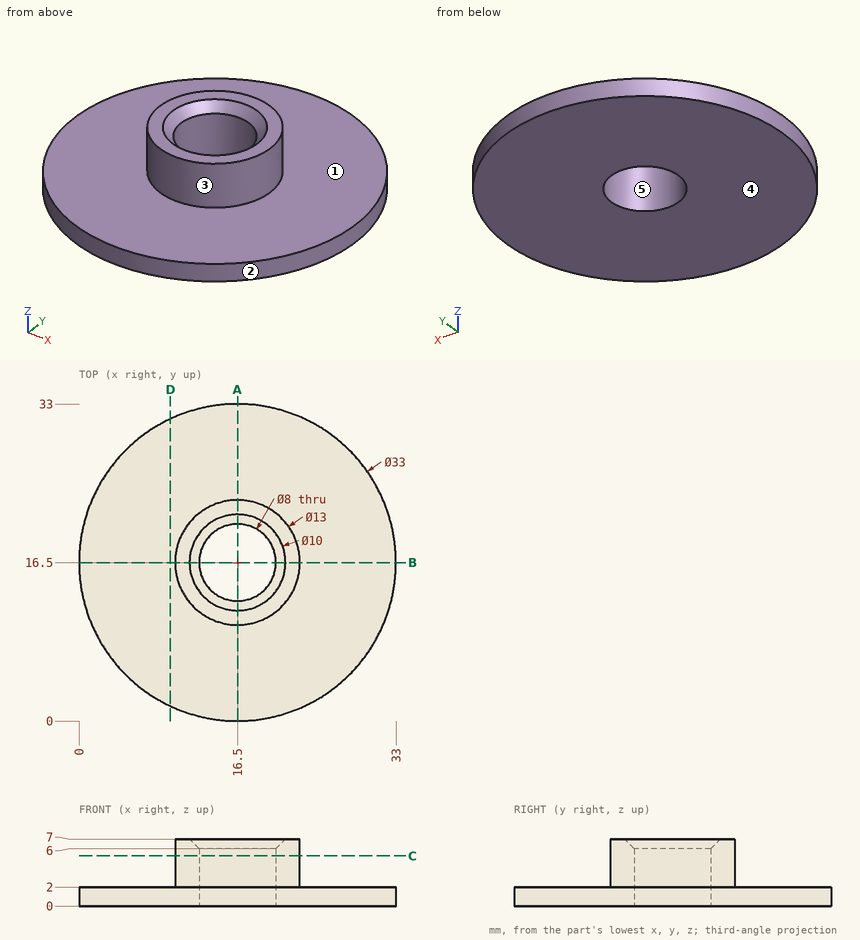
Here's the drawing with two shaded views (mm, measured from the low corner). I have some questions. A direction names the side the tool comes from. Give positions to 0.01 mm unless a question says otherwise; leave off trailing zeros. Order: outer loops, then holes, each group sorted by start corner. A loop starts at its lowest first (then second) coordinate and runs counter-clockwise, first axis right, second up. Notation, with made-up numbers: M 29,-6 L 36,-6 A33 ccw 36,28 Z; hole C 81,49.25 d8. An arc over 180 degrees is marked long. One line per item, written item: value.
1) I want a section at A-A, the plane x = 16.5. List the corners of the cut face in (y, z) for me, plus the area to 3 significant figures.
Answer sheet:
outline: M 0,0 L 12.5,0 L 12.5,6 L 11.5,7 L 10,7 L 10,2 L 0,2 Z; M 20.5,0 L 33,0 L 33,2 L 23,2 L 23,7 L 21.5,7 L 20.5,6 Z
area: 74.0 mm^2
2) I want a section at C-C, the plane z = 5.25. List the corners of the cut face in (x, y) for me.
Answer sheet:
outline: C 16.5,16.5 d13; hole C 16.5,16.5 d8
3) We'd pull the mould along X, two halves only. Please class the marked faces 3, 4 and 5: released by +X, released by -X, zero draft, split by the parting line, or undercut.
Answer sheet:
face 3: split by the parting line
face 4: zero draft
face 5: undercut
4) For P1, Ø4, axis at x = 26.5, z = 2.5, coming from the +Y side; P2, Ø3, axis at y = 25, z = 3, coming from the +X side; P3, Ø9, axis at x = 16.5, y = 16.5, coming from the +Z side, each with a flat end and sliding along its axis, tell me the tip position at first contact or that it passes through.
Answer sheet:
P1: stops at y = 30.9
P2: stops at x = 31.26
P3: stops at z = 6.5
5) Please list where these lines run through material, in increasing order: line 1 along Y through (x, z) = (16.5, 2.8); line 2 along Y through (x, z) = (16.5, 1.3); line 3 along Z through (x, y) = (21, 4.5).
Answer sheet:
line 1: y = 10 to 12.5, 20.5 to 23
line 2: y = 0 to 12.5, 20.5 to 33
line 3: z = 0 to 2
6) I want a section at D-D, the plane x = 9.5. List the corners of the cut face in (y, z) for me, plus the area to 3 significant figures.
Answer sheet:
outline: M 1.56,0 L 31.44,0 L 31.44,2 L 1.56,2 Z
area: 59.8 mm^2
7) On a 3-axis mill with a long thin cutter (end or side, diameter ignored), from which of +Z, -Z, +X, -X, +Y, -Y can I reach the whole of each face in a straight line? I mean the marked faces 1 and 2. Say none if no direction works.
Answer sheet:
face 1: +Z
face 2: +Z, -Z
